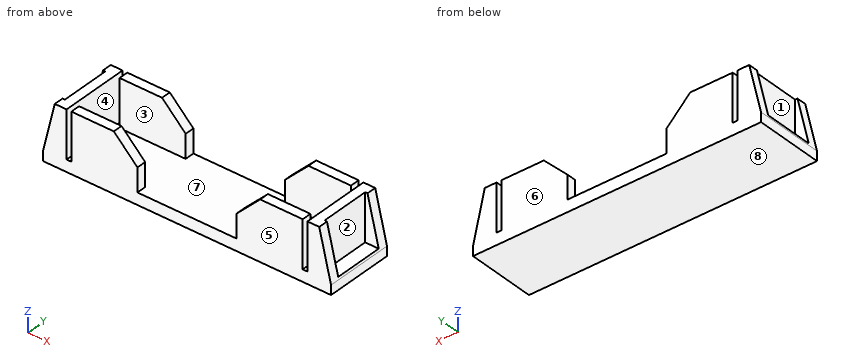
Autodesk Fusion 360 part; units mm, degrees
sketch "Sketch1" plane through (0, 0, 0) normal (0, 0, 1) x (1, 0, 0)
  line L0 (0, 0) -> (61, 0)
  line L1 (61, 0) -> (61, 14.5)
  line L2 (61, 14.5) -> (0, 14.5)
  line L3 (0, 14.5) -> (0, 0)
  dimension "d1" = 61
  dimension "d2" = 14.5
extrude "Extrude1" add sketch "Sketch1" along normal blind 2.5
sketch "Sketch2" plane through (0, 0, 2.5) normal (0, 0, 1) x (-1, 0, 0)
  line L0 (0, -14.5) -> (0, 0)
  line L1 (0, 0) -> (-61, 0)
  line L2 (-61, 0) -> (-61, -14.5)
  line L3 (-61, -14.5) -> (0, -14.5)
  line L4 (-5, -24.7983) -> (-5, 20) construction
  line L5 (-56, -25) -> (-56, 25) construction
  line L6 (12, -12.5) -> (-78, -12.5) construction
  line L7 (12, -2) -> (-79, -2) construction
  line L8 (-5, -14.5) -> (-3, -14.5)
  line L9 (-3, -14.5) -> (-3, 0)
  line L10 (-3, 0) -> (-5, 0)
  line L11 (-5, 0) -> (-5, -14.5)
  line L12 (-56, -14.5) -> (-58, -14.5)
  line L13 (-58, -14.5) -> (-58, 0)
  line L14 (-58, 0) -> (-56, 0)
  line L15 (-56, 0) -> (-56, -14.5)
  line L16 (-6, -14.5) -> (-20, -14.5)
  line L17 (-20, -14.5) -> (-20, -12.5)
  line L18 (-20, -12.5) -> (-6, -12.5)
  line L19 (-6, -12.5) -> (-6, -14.5)
  line L20 (-6, -2) -> (-20, -2)
  line L21 (-20, -2) -> (-20, 0)
  line L22 (-20, 0) -> (-6, 0)
  line L23 (-6, 0) -> (-6, -2)
  line L24 (-55, -14.5) -> (-41, -14.5)
  line L25 (-41, -14.5) -> (-41, -12.5)
  line L26 (-41, -12.5) -> (-55, -12.5)
  line L27 (-55, -12.5) -> (-55, -14.5)
  line L28 (-41, -2) -> (-55, -2)
  line L29 (-55, -2) -> (-55, 0)
  line L30 (-55, 0) -> (-41, 0)
  line L31 (-41, 0) -> (-41, -2)
  line L32 (-3, -14.5) -> (0, -14.5)
  line L33 (0, -14.5) -> (0, -12.5)
  line L34 (0, -12.5) -> (-3, -12.5)
  line L35 (-3, -12.5) -> (-3, -14.5)
  line L36 (-58, -14.5) -> (-61, -14.5)
  line L37 (-61, -14.5) -> (-61, -12.5)
  line L38 (-61, -12.5) -> (-58, -12.5)
  line L39 (-58, -12.5) -> (-58, -14.5)
  line L40 (-58, -2) -> (-61, -2)
  line L41 (-61, -2) -> (-61, 0)
  line L42 (-61, 0) -> (-58, 0)
  line L43 (-58, 0) -> (-58, -2)
  line L44 (-3, -2) -> (0, -2)
  line L45 (0, -2) -> (0, 0)
  line L46 (0, 0) -> (-3, 0)
  line L47 (-3, 0) -> (-3, -2)
  dimension "d5" = 51
  dimension "d6" = 5
  dimension "d7" = 10.5
  dimension "d8" = 2
  dimension "d9" = 14
  dimension "d10" = 14
  dimension "d11" = 14
  dimension "d12" = 14
  dimension "d13" = 1
  dimension "d14" = 1
  dimension "d15" = 1
  dimension "d16" = 1
extrude "Extrude2" add sketch "Sketch2" along normal blind 10 contours L0 L3 L9 L32 L33 L34 L35 | L1 L3 L8 L9 L10 L11 L35 L47 | L0 L1 L9 L44 L45 L46 L47 | L3 L16 L17 L18 L19 | L1 L20 L21 L22 L23 | L3 L24 L25 L26 L27 | L1 L28 L29 L30 L31 | L1 L3 L12 L13 L14 L15 L39 L43 | L2 L3 L13 L36 L37 L38 L39 | L1 L2 L13 L40 L41 L42 L43
sketch "Sketch3" plane through (0, 0, 0) normal (0, -1, 0) x (1, 0, 0)
  line L0 (0, 0) -> (61, 0)
  line L1 (61, 0) -> (61, 12.5)
  line L2 (61, 12.5) -> (56, 12.5)
  line L3 (56, 12.5) -> (56, 2.5)
  line L4 (56, 2.5) -> (55, 2.5)
  line L5 (55, 2.5) -> (55, 12.5)
  line L6 (55, 12.5) -> (41, 12.5)
  line L7 (41, 12.5) -> (41, 2.5)
  line L8 (41, 2.5) -> (20, 2.5)
  line L9 (20, 2.5) -> (20, 12.5)
  line L10 (20, 12.5) -> (6, 12.5)
  line L11 (6, 12.5) -> (6, 2.5)
  line L12 (6, 2.5) -> (5, 2.5)
  line L13 (5, 2.5) -> (5, 12.5)
  line L14 (5, 12.5) -> (0, 12.5)
  line L15 (0, 12.5) -> (0, 0)
  line L16 (2.5, 12.5) -> (0, 2)
  line L17 (0, 12.5) -> (0, 2)
  line L18 (0, 12.5) -> (2.5, 12.5)
  line L19 (58.5, 12.5) -> (61, 2)
  line L20 (61, 2) -> (61, 12.5)
  line L21 (61, 12.5) -> (58.5, 12.5)
extrude "Extrude3" cut sketch "Sketch3" against normal blind 68 contours L14 L15 L16 L17 L18 | L1 L2 L19 L20 L21
chamfer "Chamfer1" distance 5 angle 45 4 edges at (20, 13.5, 12.5) (41, 13.5, 12.5) (41, 1, 12.5) (20, 1, 12.5)
Read the model definition and answer for the solid it produces. Units are mm, in the model's axes. Face numbers are marked on the shaded views. A direction names the side the tool comes from. Round coordinates to 2 decimals unless told otherwise and drop trailing zeros. Write each loop counter-clockwise with the first axis right and the second up, starting at its lowest first coordinate (ties: lowest second). Pieces come first, ordered by that corner, then holes. Notation, with made-up numbers: (-2, 87) -> (24, 87) arc R13 ccw to (24, 94) -> close; hole circle Ø11 at (-9, 41). An arc over 180 degrees is marked (long way). Answer in a Markdown table with one row per item. Add a question column.
1) Find section A-A, the plane y = 10.5. Determine the outline of the cut face in (x, z).
2) Find section B-B, the plane x = 8.5. Determine the outline of the cut face in (y, z).
3) Determine the mould class of the marked faces 6, 7 and 8 for opening direction Y: pulls with the +Y half, pulls with the -Y half, needs draft (parallel to the pull), parting line crosses it, or undercut.
4) Find section C-C, the plane z = 5. State how many separate pieces and enclosed holes the cut face has, and give its area (3 significant figures).
5) Find section D-D, the plane y = 13.25. Determine the outline of the cut face in (x, z), and give its area (3 significant figures).
6) Given P1, Ø0.6, axis at y = 13, z = 9, coming from the +X side; P2, Ø2, axis at x = 7, y = 7.5, coming from the +Z side; P3, Ø0.6, axis at y = 1, z = 10, coming from the -X side, each flat-ended and moving along its own axis, determine where each tip first touches the part or whether it passes through.
7) Consider line 1 (X direction, y = 11.25, z = 4.75); line 2 (X direction, y = 0.5, z = 6.5); line 3 (Y direction, x = 8, z = 12). Determine where each line is inside the solid, lowest interval first.
8) Which of the six approach directions +Z, -Z, +X, -X, +Y, -Y give full straight-line access (tool end or side, diameter ignored) to the marked faces 1, 2, 3, 4 and 5?
Findings below:
| question | item | result |
|---|---|---|
| 1 | outline | (0, 0) -> (61, 0) -> (61, 2) -> (60.88, 2.5) -> (58, 2.5) -> (58, 12.5) -> (56, 12.5) -> (56, 2.5) -> (5, 2.5) -> (5, 12.5) -> (3, 12.5) -> (3, 2.5) -> (0.12, 2.5) -> (0, 2) -> close |
| 2 | outline | (0, 0) -> (14.5, 0) -> (14.5, 12.5) -> (12.5, 12.5) -> (12.5, 2.5) -> (2, 2.5) -> (2, 12.5) -> (0, 12.5) -> close |
| 3 | face 6 | pulls with the +Y half |
| 3 | face 7 | undercut |
| 3 | face 8 | needs draft |
| 4 | separate pieces | 6 |
| 4 | enclosed holes | 0 |
| 4 | area | 188 mm² |
| 5 | outline | (0, 0) -> (61, 0) -> (61, 2) -> (58.5, 12.5) -> (56, 12.5) -> (56, 2.5) -> (55, 2.5) -> (55, 12.5) -> (46, 12.5) -> (41, 7.5) -> (41, 2.5) -> (20, 2.5) -> (20, 7.5) -> (15, 12.5) -> (6, 12.5) -> (6, 2.5) -> (5, 2.5) -> (5, 12.5) -> (2.5, 12.5) -> (0, 2) -> close |
| 5 | area | 481 mm² |
| 6 | P1 | x = 59.4 |
| 6 | P2 | z = 2.5 |
| 6 | P3 | x = 1.83 |
| 7 | line 1 | 3 to 5, 56 to 58 |
| 7 | line 2 | 1.07 to 5, 6 to 20, 41 to 55, 56 to 59.93 |
| 7 | line 3 | 0 to 2, 12.5 to 14.5 |
| 8 | face 1 | +Z, -X |
| 8 | face 2 | +Z, +X |
| 8 | face 3 | +Z |
| 8 | face 4 | +Z, +Y, -Y |
| 8 | face 5 | +Z, -Z, +X, -X, -Y |
